Verification items for the finished model (mm, model axes). A direction names the side the tool comes from. Round coordinates to 2 decimals unless told otherwise and drop trailing zeros. Write each loop counter-clockwise with the first axis right and the second up, starting at its lowest first coordinate (ties: lowest second). Pieces come first, ordered by that corner, then holes. Notation, with made-up numbers: (56, 83.5) - (80, 83.5) arc R37 ccw to (80, 119.5) - close; hole circle Ø11 at (44, 17.25). An arc over 180 degrees is marked (long way). Answer as a JSON object with one key per item and string values.
```python
from build123d import *

# Parameters (mm, degrees)
ESQUISSE1_W             = 38
ESQUISSE1_H             = 25
BOSS_EXTRU_1_DEPTH      = 6
ENL_V_MAT_EXTRU_1_DEPTH = 6
BOSS_EXTRU_2_DEPTH      = 6
ESQUISSE4_R             = 2.052376102
ENL_V_MAT_EXTRU_2_DEPTH = 6
CHANFREIN2_SIZE         = 4


with BuildPart() as part:
    # Esquisse1 → Boss.-Extru.1 (new body)
    with BuildSketch(Plane.XY):
        Rectangle(ESQUISSE1_W, ESQUISSE1_H)
    extrude(amount=BOSS_EXTRU_1_DEPTH)

    # Esquisse2 → Enlèv. mat.-Extru.1 (cut)
    with BuildSketch(Plane.XY.offset(6)):
        Polygon((2.5, 12.5), (-2.5, 12.5), (-2.5, 7.5), (-4.3, 7.5), (-4.3, 2), (-2.5, 2), (-2.5, -2), (2.5, -2), (2.5, 2), (4.3, 2), (4.3, 7.5), (2.5, 7.5), align=None)
    extrude(amount=-ENL_V_MAT_EXTRU_1_DEPTH, mode=Mode.SUBTRACT)

    # Esquisse2<3> → Boss.-Extru.2 (add)
    with BuildSketch(Plane.XY.offset(6)):
        with BuildLine():
            Line((-15.5, 17.5), (-15.5, 12.5))
            Line((-15.5, 12.5), (-7.5, 12.5))
            Line((-7.5, 12.5), (-7.5, 17.5))
            ThreePointArc((-7.5, 17.5), (-7.792893219, 18.207106781), (-8.5, 18.5))
            Line((-8.5, 18.5), (-14.5, 18.5))
            ThreePointArc((-14.5, 18.5), (-15.207106781, 18.207106781), (-15.5, 17.5))
        make_face()
        with BuildLine():
            Line((7.5, 17.5), (7.5, 12.5))
            Line((7.5, 12.5), (15.5, 12.5))
            Line((15.5, 12.5), (15.5, 17.5))
            ThreePointArc((15.5, 17.5), (15.207106781, 18.207106781), (14.5, 18.5))
            Line((14.5, 18.5), (8.5, 18.5))
            ThreePointArc((8.5, 18.5), (7.792893219, 18.207106781), (7.5, 17.5))
        make_face()
    extrude(amount=-BOSS_EXTRU_2_DEPTH)

    # Esquisse4 → Enlèv. mat.-Extru.2 (cut)
    with BuildSketch(Plane.XY.offset(6)):
        with Locations((-12, -2.5)):
            Circle(ESQUISSE4_R)
    enl_v_mat_extru_2 = extrude(amount=-ENL_V_MAT_EXTRU_2_DEPTH, mode=Mode.SUBTRACT)

    # Symétrie7: Enlèv. mat.-Extru.2 across plane
    add(enl_v_mat_extru_2.mirror(Plane(origin=(0, 0, 0), x_dir=(0, 0, 1), z_dir=(1, 0, 0))), mode=Mode.SUBTRACT)

    # Chanfrein2
    chanfrein2_edges = [part.edges().sort_by_distance(p)[0] for p in [
        (19, -12.5, 3),
        (-19, -12.5, 3),
    ]]
    chamfer(chanfrein2_edges, length=CHANFREIN2_SIZE)


solid = part.part
```
1. Cross-section at A-A (x = -3). Record the boundary of the cut face in (y, z).
Completed:
{"outline": "(-12.5, 0) - (2, 0) - (2, 6) - (-12.5, 6) - close; (7.5, 0) - (12.5, 0) - (12.5, 6) - (7.5, 6) - close"}
2. Cross-section at B-B (y = -2.5). Record the boundary of the cut face in (x, z), plus the area to 3 significant figures.
Completed:
{"outline": "(-19, 0) - (-14.05, 0) - (-14.05, 6) - (-19, 6) - close; (-9.95, 0) - (9.95, 0) - (9.95, 6) - (-9.95, 6) - close; (14.05, 0) - (19, 0) - (19, 6) - (14.05, 6) - close", "area": "179 mm^2"}
3. Cross-section at D-D (z = 0.5). Count the separate pieces of the cut face and the enclosed holes in it, plus the area to 3 significant figures.
Completed:
{"separate pieces": "1", "enclosed holes": "2", "area": "910 mm^2"}
4. Material ranges on probe 1 along X at (y, z) = (4, 1.75); probe 2 along X at (y, z) = (10, 3.5); probe 3 along Y at (x, z) = (-12, 3.95), recorded low to high. Write a range as from..to.
Completed:
{"probe 1": "x = -19..-4.3, 4.3..19", "probe 2": "x = -19..-2.5, 2.5..19", "probe 3": "y = -12.5..-4.55, -0.45..18.5"}
5. Mould release check, pull along X, two halves, no side actions. Record for faces 1 (the face through (-11, 18.5, 3)), 2 (the face through (15.5, 15, 3)), 3 (the face through (-17, -10.5, 3)), 4 (the face through (0, -2, 3)): released by +X, released by -X, zero draft, split by the parting line, or undercut.
Completed:
{"face 1": "zero draft", "face 2": "released by +X", "face 3": "released by -X", "face 4": "undercut"}
6. Access from +Z, -Z, +X, -X, +Y, -Y to the whole of each face (thin tool, end or side, straight path). Record for faces 5 (the face through (-15.5, 15, 3)), 6 (the face through (-3, 2, 3)), 7 (the face through (17, 12.5, 3)), 8 (the face through (-7.5, 15, 3)).
Completed:
{"face 5": "+Z, -Z, -X, +Y", "face 6": "+Z, -Z", "face 7": "+Z, -Z, +X, +Y", "face 8": "+Z, -Z, +Y"}
7. Cross-section at C-C (y = 3). Record the boundary of the cut face in (x, z).
Completed:
{"outline": "(-19, 0) - (-4.3, 0) - (-4.3, 6) - (-19, 6) - close; (4.3, 0) - (19, 0) - (19, 6) - (4.3, 6) - close"}
8. Go/stop test with flat-tipped pins: pin 1 (2.5 mm diameter, centred on x = 0.5, z = 4, fed in from +Y); pin 2 (0.9 mm diameter, centred on x = 3.5, z = 3, fed in from +Y); pin 3 (1.5 mm diameter, centred on y = 14, z = 2, fed in from +X). Record where each tip stops, or that it passes through.
Completed:
{"pin 1": "stops at y = -2", "pin 2": "stops at y = 12.5", "pin 3": "stops at x = 15.5"}
